Part model, mm, in its own coordinate system. A direction names the side the tool comes from. Round coordinates to 2 decimals unless told otherwise and drop trailing zeros. Write each loop counter-clockwise with the first axis right and the second up, starting at its lowest first coordinate (ties: lowest second). Pieces come first, ordered by that corner, then holes.
```python
from build123d import *

# Parameters (mm, degrees)
SKETCH3_R          = 1
CUT_EXTRUDE1_DEPTH = 10
SKETCH4_R          = 1
CUT_EXTRUDE2_DEPTH = 10


with BuildPart() as part:
    # Sketch1 → Revolve1 (revolve)
    with BuildSketch(Plane.XY):
        Polygon((2.5, 0), (5, 0), (5, 5), (4, 5), (4, 15), (5, 15), (5, 17), (2.5, 17), align=None)
    revolve(axis=Axis((0, 0, 0), (0, 1, 0)))

    # Sketch3 → Cut-Extrude1 (cut)
    with BuildSketch(Plane.XY):
        with Locations((0, 2.5)):
            Circle(SKETCH3_R)
    extrude(amount=-CUT_EXTRUDE1_DEPTH, mode=Mode.SUBTRACT)

    # Sketch4 → Cut-Extrude2 (cut)
    with BuildSketch(Plane(origin=(0, 0, 0), x_dir=(0, 0, -1), z_dir=(1, 0, 0))):
        with Locations((0, 2.5)):
            Circle(SKETCH4_R)
    extrude(amount=-CUT_EXTRUDE2_DEPTH, mode=Mode.SUBTRACT)


solid = part.part
```
Q1. Cut at B-B on z = 0. Write the cut outline in (x, y), plus the area to 3 significant figures.
Values follow:
outline: (-5, 0) - (-2.5, 0) - (-2.5, 1.5) - (-5, 1.5) - close; (-5, 3.5) - (-2.5, 3.5) - (-2.5, 17) - (-5, 17) - (-5, 15) - (-4, 15) - (-4, 5) - (-5, 5) - close; (2.5, 0) - (5, 0) - (5, 5) - (4, 5) - (4, 15) - (5, 15) - (5, 17) - (2.5, 17) - close
area: 60.0 mm2
Q2. Which spindle directions (+Z, -Z, +X, -X, +Y, -Y) get a long thin tool onto all of the face, cutting with end or side? Do faces 4 (the cylindrical face through (-1, 2.5, -3.6)), 5 (the cylindrical face through (2.307, 2.535, 4.436)), 6 (the cylindrical face through (-3.6, 2.5, 1)). Say none if no direction does.
Values follow:
face 4: -Z
face 5: +Y, -Y
face 6: -X
Q3. Wall check: L1, parallel to Z at x = 0, y = 15.75; L2, parallel to Y at x = 0, z = -3.4. Give the ranges that are in metal, low to high.
Values follow:
L1: z = -5 to -2.5, 2.5 to 5
L2: y = 0 to 1.5, 3.5 to 17
Q4. Drop flat-ended pins along their axis: pin 1 (1.5 mm diameter, centred on x = 4, y = 3.5, fed in from -Z); pin 2 (2.5 mm diameter, centred on x = 0, y = 2.5, fed in from -Z); pin 3 (1.8 mm diameter, centred on y = 2.5, z = 0, fed in from -X); pin 4 (2 mm diameter, centred on x = -1.5, y = 10.5, fed in from -Z). Give the stop position or say it passes through.
Values follow:
pin 1: stops at z = -3.8
pin 2: stops at z = -5
pin 3: stops at x = 2.33
pin 4: stops at z = -3.97
Q5. Cut at D-D on z = -1.25. Write the cut outline in (x, y).
Values follow:
outline: (-4.84, 0) - (-2.17, 0) - (-2.17, 17) - (-4.84, 17) - (-4.84, 15) - (-3.8, 15) - (-3.8, 5) - (-4.84, 5) - close; (2.17, 0) - (4.84, 0) - (4.84, 5) - (3.8, 5) - (3.8, 15) - (4.84, 15) - (4.84, 17) - (2.17, 17) - close
Q6. Cut at A-A on x = 0. Write the cut outline in (y, z), plus the area to 3 significant figures.
Values follow:
outline: (0, -5) - (1.5, -5) - (1.5, -2.5) - (0, -2.5) - close; (0, 2.5) - (17, 2.5) - (17, 5) - (15, 5) - (15, 4) - (5, 4) - (5, 5) - (0, 5) - close; (3.5, -5) - (5, -5) - (5, -4) - (15, -4) - (15, -5) - (17, -5) - (17, -2.5) - (3.5, -2.5) - close
area: 60.0 mm2
Q7. Cut at C-C on y = 2.5. Write the cut outline in (x, z), plus the area to 3 significant figures.
Values follow:
outline: (-4.9, -1) arc R5 ccw to (-1, -4.9) - (-1, -2.29) arc R2.5 cw to (-2.29, -1) - close; (-4.9, 1) - (-2.29, 1) arc R2.5 cw (long way) to (1, -2.29) - (1, -4.9) arc R5 ccw (long way) to start
area: 48.8 mm2
Q8. Mould opens along Y. For faces 1 (the flat face through (2, 17, 2)), 2 (the flat face through (-2, 0, 2)), 3 (the cylindrical face through (-0.867, 10.07, 3.905)) say: +Y half, -Y half, draft (parallel to the pull), parting line (faces both ways), or undercut.
Values follow:
face 1: +Y half
face 2: -Y half
face 3: undercut
